from build123d import *

# Parameters (mm, degrees)
SKETCH_2_W          = 44
SKETCH_2_H          = 72.5
EXTRUDE_1_DEPTH     = 59.4
SKETCH_3_R          = 1.75
CUT_EXTRUDE_1_DEPTH = 60.4
SKETCH_4_W          = 39.4
SKETCH_4_H          = 31.25
CUT_EXTRUDE_2_DEPTH = 45
FILLET_1_R          = 2


with BuildPart() as part:
    # ｽｹｯﾁ2 → ﾎﾞｽ - 押し出し1 (new body)
    with BuildSketch(Plane.XY):
        Rectangle(SKETCH_2_W, SKETCH_2_H)
    extrude(amount=EXTRUDE_1_DEPTH)

    # ｽｹｯﾁ3 → ｶｯﾄ - 押し出し1 (cut, through all)
    with BuildSketch(Plane.XY.offset(59.4)):
        with Locations((-16, 31.25)):
            Circle(SKETCH_3_R)
        with Locations((16, 31.25)):
            Circle(SKETCH_3_R)
        with Locations((16, -31.25)):
            Circle(SKETCH_3_R)
        with Locations((-16, -31.25)):
            Circle(SKETCH_3_R)
    extrude(amount=-CUT_EXTRUDE_1_DEPTH, mode=Mode.SUBTRACT)

    # ｽｹｯﾁ4 → ｶｯﾄ - 押し出し2 (cut, through all)
    with BuildSketch(Plane(origin=(22, 0, 0), x_dir=(0, 0, -1), z_dir=(1, 0, 0))):
        with Locations((-29.7, -20.625)):
            Rectangle(SKETCH_4_W, SKETCH_4_H)
        with Locations((-29.7, 20.625)):
            Rectangle(SKETCH_4_W, SKETCH_4_H)
    extrude(amount=-CUT_EXTRUDE_2_DEPTH, mode=Mode.SUBTRACT)

    # ﾌｨﾚｯﾄ1
    fillet_1_edges = [part.edges().sort_by_distance(p)[0] for p in [
        (22, -36.25, 5),
        (-22, -36.25, 5),
        (-22, 36.25, 5),
        (22, 36.25, 5),
        (-22, 36.25, 54.4),
        (22, 36.25, 54.4),
        (22, -36.25, 54.4),
        (-22, -36.25, 54.4),
    ]]
    fillet(fillet_1_edges, radius=FILLET_1_R)


solid = part.part
Check sheet for the modelled part. Datum: model origin and axes. Units: mm. A direction names the side the tool comes from. Round coordinates to 2 decimals unless told otherwise and drop trailing zeros. Loops run counter-clockwise (first coordinate to the right, second up) from the corner with the lowest first, then second, coordinate; pieces in that order, holes last.
1. Sectioned sample at B-B on x = 16. Record the boundary of the cut face in (y, z).
2. Sectioned sample at D-D on x = -13. Record the boundary of the cut face in (y, z), and give its area (3 significant figures).
3. Sectioned sample at A-A on y = -31.25. Record the boundary of the cut face in (x, z).
4. Set-up check for faces 5 (the cylindrical face through (16.941, 32.726, 54.47)), 6 (the flat face through (0, -21, 10)): record each of +Z, -Z, +X, -X, +Y, -Y from which the full face is reachable in a straight line by a thin tool's end or side.
5. Scan lines: probe 1 along X at (y, z) = (-31, 6); probe 2 along Y at (x, z) = (16, 55); probe 3 along Z at (x, y) = (2.5, -14). Record each from-to range of solid material in increasing order.
6. Gauge pin test, flat ends, axial feed: pin 1 Ø19.5 at (x, z) = (-6.5, 23.5) entering from -Y; pin 2 Ø3 at (x, y) = (-16, 31.25) entering from -Z; pin 3 Ø12 at (x, z) = (4, 36.5) entering from +Y. Record the tip position at first contact, or that the pin passes through.
7. Mould release check, pull along Z, two halves, no side actions. Record for faces 1 (the flat face through (0, -5, 30)), 2 (the flat face through (0, 20, 10)), 3 (the cylindrical face through (21.4, -35.68, 5.07)), 4 (the flat face through (0, 1, 0)): released by +Z, released by -Z, zero draft, split by the parting line, or undercut.
8. Sectioned sample at C-C on y = 13. Record the boundary of the cut face in (x, z), and give its area (3 significant figures).
Recorded:
1. outline: (-36.25, 0) - (-33, 0) - (-33, 10) - (-36.25, 10) - close; (-36.25, 49.4) - (-33, 49.4) - (-33, 59.4) - (-36.25, 59.4) - close; (-29.5, 0) - (29.5, 0) - (29.5, 10) - (5, 10) - (5, 49.4) - (29.5, 49.4) - (29.5, 59.4) - (-29.5, 59.4) - (-29.5, 49.4) - (-5, 49.4) - (-5, 10) - (-29.5, 10) - close; (33, 0) - (36.25, 0) - (36.25, 10) - (33, 10) - close; (33, 49.4) - (36.25, 49.4) - (36.25, 59.4) - (33, 59.4) - close
2. outline: (-36.25, 0) - (36.25, 0) - (36.25, 10) - (5, 10) - (5, 49.4) - (36.25, 49.4) - (36.25, 59.4) - (-36.25, 59.4) - (-36.25, 49.4) - (-5, 49.4) - (-5, 10) - (-36.25, 10) - close
2. area: 1,840 mm2
3. outline: (-22, 0) - (-17.75, 0) - (-17.75, 10) - (-22, 10) - close; (-22, 49.4) - (-17.75, 49.4) - (-17.75, 59.4) - (-22, 59.4) - close; (-14.25, 0) - (14.25, 0) - (14.25, 10) - (-14.25, 10) - close; (-14.25, 49.4) - (14.25, 49.4) - (14.25, 59.4) - (-14.25, 59.4) - close; (17.75, 0) - (22, 0) - (22, 10) - (17.75, 10) - close; (17.75, 49.4) - (22, 49.4) - (22, 59.4) - (17.75, 59.4) - close
4. face 5: +Z, -Z
4. face 6: +X, -X, -Y
5. probe 1: x = -22 to -17.73, -14.27 to 14.27, 17.73 to 22
5. probe 2: y = -36.25 to -33, -29.5 to 29.5, 33 to 36.25
5. probe 3: z = 0 to 10, 49.4 to 59.4
6. pin 1: stops at y = -5
6. pin 2: passes through
6. pin 3: stops at y = 5
7. face 1: undercut
7. face 2: undercut
7. face 3: zero draft
7. face 4: released by -Z
8. outline: (-22, 0) - (22, 0) - (22, 10) - (-22, 10) - close; (-22, 49.4) - (22, 49.4) - (22, 59.4) - (-22, 59.4) - close
8. area: 880 mm2
